from build123d import *

# Parameters (mm, degrees)
SKETCH_1_R          = 2.835000467
SKETCH_1_R_2        = 2.835
EXTRUDE_1_DEPTH     = 5
CUT_EXTRUDE_START   = -5
CUT_EXTRUDE_1_DEPTH = 5


with BuildPart() as part:
    # Эскиз1 → Бобышка-Вытянуть1 (new body)
    with BuildSketch(Plane(origin=(0, 0, 0), x_dir=(0, 0, -1), z_dir=(1, 0, 0))):
        with BuildLine():
            Line((-4.835001402, 17.999999558), (-4.835001402, -18.000000151))
            ThreePointArc((-4.835001402, -18.000000151), (-9.35e-07, -22.835000618), (4.834999533, -18.000000151))
            Line((4.834999533, -18.000000151), (4.834999533, 17.999999558))
            ThreePointArc((4.834999533, 17.999999558), (-9.35e-07, 22.835000025), (-4.835001402, 17.999999558))
        make_face()
        with Locations((0, 17.999999684)):
            Circle(SKETCH_1_R, mode=Mode.SUBTRACT)
        with Locations((-3.97e-07, 5.999999684)):
            Circle(SKETCH_1_R_2, mode=Mode.SUBTRACT)
        with Locations((-4.67e-07, -6.000000151)):
            Circle(SKETCH_1_R_2, mode=Mode.SUBTRACT)
        with Locations((-4.67e-07, -18.000000151)):
            Circle(SKETCH_1_R_2, mode=Mode.SUBTRACT)
    extrude(amount=EXTRUDE_1_DEPTH)

    # Эскиз2 → Вырез-Вытянуть1 (cut)
    with BuildSketch(Plane(origin=(5, 0, 0), x_dir=(0, 0, -1), z_dir=(1, 0, 0)).offset(CUT_EXTRUDE_START)):
        with BuildLine():
            Line((-4.835001402, 17.999999558), (-4.835001402, -18.000000151))
            ThreePointArc((-4.835001402, -18.000000151), (-9.35e-07, -22.835000618), (4.834999533, -18.000000151))
            Line((4.834999533, -18.000000151), (4.834999533, 17.999999558))
            ThreePointArc((4.834999533, 17.999999558), (-9.35e-07, 22.835000025), (-4.835001402, 17.999999558))
        make_face()
        with BuildLine():
            Line((-4.335001402, 17.999999558), (-4.335001402, -18.000000151))
            ThreePointArc((-4.335001402, -18.000000151), (-9.35e-07, -22.335000618), (4.334999533, -18.000000151))
            Line((4.334999533, -18.000000151), (4.334999533, 17.999999558))
            ThreePointArc((4.334999533, 17.999999558), (-9.35e-07, 22.335000025), (-4.335001402, 17.999999558))
        make_face(mode=Mode.SUBTRACT)
    extrude(amount=CUT_EXTRUDE_1_DEPTH, mode=Mode.SUBTRACT)


solid = part.part
Read the model definition and answer for the solid it produces. Units are mm, in the model's axes. Coordinates: 2 decimals unless noted, no trailing zeros. Loops run counter-clockwise (first coordinate to the right, second up) from the corner with the lowest first, then second, coordinate; pieces in that order, holes last. Notation, with made-up numbers: (27.5, 70.25) -> (34.5, 70.25) arc R12 ccw to (34.5, 74.25) -> close; hole circle Ø1 at (6, 32). An arc over 180 degrees is marked (long way). Write item = value, one per line. Start each with the question number.
1) The part is cut by section D-D, the plane z = 2. Determine the outline of the cut face in (x, y), plus the area to 3 significant figures.
2) Given P1, Ø1, axis at x = 2.5, z = -2, coming from the -Y side, flat-ended and moving along its own axis, determine where the tip first touches the part or whether it passes through.
3) The part is cut by section A-A, the plane z = 0. Determine the outline of the cut face in (x, y) (3 decimals).
4) The mould has two halves that part along Z. Classify faces 1 (the face through (2.46, -3.19, 0.37)), 2 (the face through (2.465, -22.334, 0.095)), 3 (the face through (2.46, 8.81, 0.37)), 4 (the face through (0, 0, 0)): pulls with the +Z half, pulls with the -Z half, needs draft (parallel to the pull), parting line crosses it, or undercut.
5) Find the intervals of material crossed by L1, parallel to Y at x = 1.3, z = 0 (3 decimals); L2, parallel to Z at x = 0.4, y = 18 (3 decimals); L3, parallel to Y at x = 3.85, z = -1.5, in increasing order. Write a range as from..to.
6) The part is cut by section C-C, the plane x = 4.6. Determine the outline of the cut face in (y, z) (3 decimals).
7) The part is cut by section B-B, the plane y = 6. Determine the outline of the cut face in (x, z) (3 decimals), plus the area to 3 significant figures.
Result:
q1.outline = (0, -21.85) -> (5, -21.85) -> (5, -20.01) -> (0, -20.01) -> close; (0, -15.99) -> (5, -15.99) -> (5, -8.01) -> (0, -8.01) -> close; (0, -3.99) -> (5, -3.99) -> (5, 3.99) -> (0, 3.99) -> close; (0, 8.01) -> (5, 8.01) -> (5, 15.99) -> (0, 15.99) -> close; (0, 20.01) -> (5, 20.01) -> (5, 21.85) -> (0, 21.85) -> close
q1.area = 138 mm²
q2.P1 = -22.07
q3.outline = (0, -22.335) -> (5, -22.335) -> (5, -20.835) -> (0, -20.835) -> close; (0, -15.165) -> (5, -15.165) -> (5, -8.835) -> (0, -8.835) -> close; (0, -3.165) -> (5, -3.165) -> (5, 3.165) -> (0, 3.165) -> close; (0, 8.835) -> (5, 8.835) -> (5, 15.165) -> (0, 15.165) -> close; (0, 20.835) -> (5, 20.835) -> (5, 22.335) -> (0, 22.335) -> close
q4.face_1 = undercut
q4.face_2 = parting line crosses it
q4.face_3 = undercut
q4.face_4 = needs draft
q5.L1 = -22.335..-20.835, -15.165..-8.835, -3.165..3.165, 8.835..15.165, 20.835..22.335
q5.L2 = -4.335..-2.835, 2.835..4.335
q5.L3 = -22.07..-20.41, -15.59..-8.41, -3.59..3.59, 8.41..15.59, 20.41..22.07
q6.outline = (-18, -4.335) -> (18, -4.335) arc R4.335 ccw to (18, 4.335) -> (-18, 4.335) arc R4.335 ccw to start; hole circle Ø5.67 at (-18, 0); hole circle Ø5.67 at (-6, 0); hole circle Ø5.67 at (6, 0); hole circle Ø5.67 at (18, 0)
q7.outline = (0, -4.335) -> (5, -4.335) -> (5, -2.835) -> (0, -2.835) -> close; (0, 2.835) -> (5, 2.835) -> (5, 4.335) -> (0, 4.335) -> close
q7.area = 15.0 mm²
